Design review of the part shown in the three views and the two pictorial views. Dimensions are in mm from the part's minimum x, y and z. Round coordinates to 2 decimals unless told otherwise and drop trailing zeros. Loops run counter-clockwise (first coordinate to the right, second up) from the corner with the lowest first, then second, coordinate; pieces in that order, holes last. Notation, with made-up numbers: M 86,53 L 130,53 A24 ccw 130,89 Z; hole C 5,69 d10. An arc over 180 degrees is marked long. Return JSON: item names as keys, results as strings. Group by question number.
Q1. To check wall thickness, follow line 1 along X through (y, z) = (1.9, 24.5); line 2 along Z through (x, y) = (18, 2.9); line 3 along Z through (x, y) = (35.5, 2.35). State the ranges of each line that lie inside material, in increasing order.
Q2. Consider section D-D (x = 14). State the section outline as (y, z) points (1 decimal).
Q3. Consider section B-B (y = 2.6). Count the separate pieces of the cut face and the enclosed holes in it, and give its area (3 significant figures).
Q4. Consider section C-C (x = 47). State the section outline as (y, z) points (1 decimal).
Q5. Clearance check with a flat-ended pin moving along its axis: pin 1 Ø1 at (y, z) = (1, 8.5) entering from +X. State where the tip first meets the part, or that it passes through.
Q6. Consider section A-A (z = 6.35). State the section outline as (x, y) points (1 decimal).
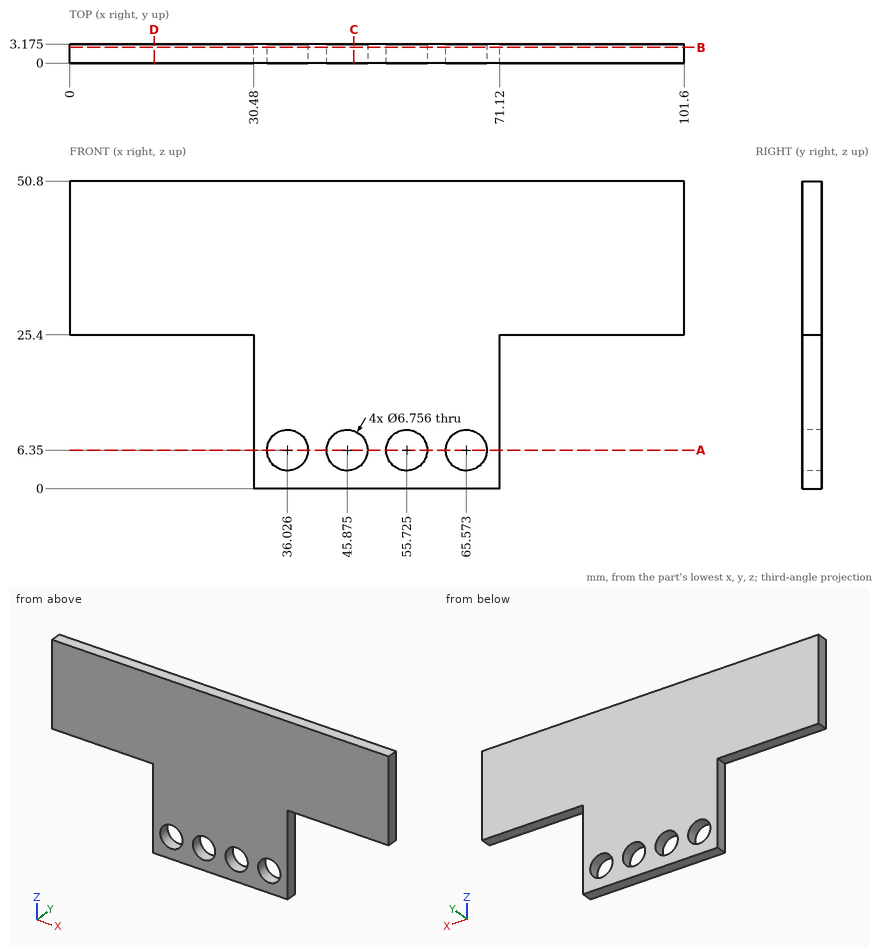
Values:
{
 "1": {"line 1": "x = 30.48 to 71.12", "line 2": "z = 25.4 to 50.8", "line 3": "z = 0 to 3.01, 9.69 to 50.8"},
 "2": {"outline": "M 0,25.4 L 3.2,25.4 L 3.2,50.8 L 0,50.8 Z"},
 "3": {"separate pieces": "1", "enclosed holes": "4", "area": "3,470 mm2"},
 "4": {"outline": "M 0,0 L 3.2,0 L 3.2,3.2 L 0,3.2 Z; M 0,9.5 L 3.2,9.5 L 3.2,50.8 L 0,50.8 Z"},
 "5": {"pin 1": "stops at x = 71.12"},
 "6": {"outline": "M 30.5,0 L 32.6,0 L 32.6,3.2 L 30.5,3.2 Z; M 39.4,0 L 42.5,0 L 42.5,3.2 L 39.4,3.2 Z; M 49.3,0 L 52.3,0 L 52.3,3.2 L 49.3,3.2 Z; M 59.1,0 L 62.2,0 L 62.2,3.2 L 59.1,3.2 Z; M 69,0 L 71.1,0 L 71.1,3.2 L 69,3.2 Z"}
}
